Verification items for this drawing (mm, ordinates from the low corner). A direction names the side the tool comes from. Give positions to 0.01 mm unless a question says otherwise; leave off trailing zeros. Order: outer loops, then holes, each group sorted by start corner. A loop starts at its lowest first (then second) coordinate and runs counter-clockwise, first axis right, second up. Notation, with made-up numbers: M 78,49.5 L 83,49.5 A26 cw 83,64.5 Z; hole C -14,84 d9. An arc over 180 degrees is marked long. Answer as a JSON object with one key per item and string values.
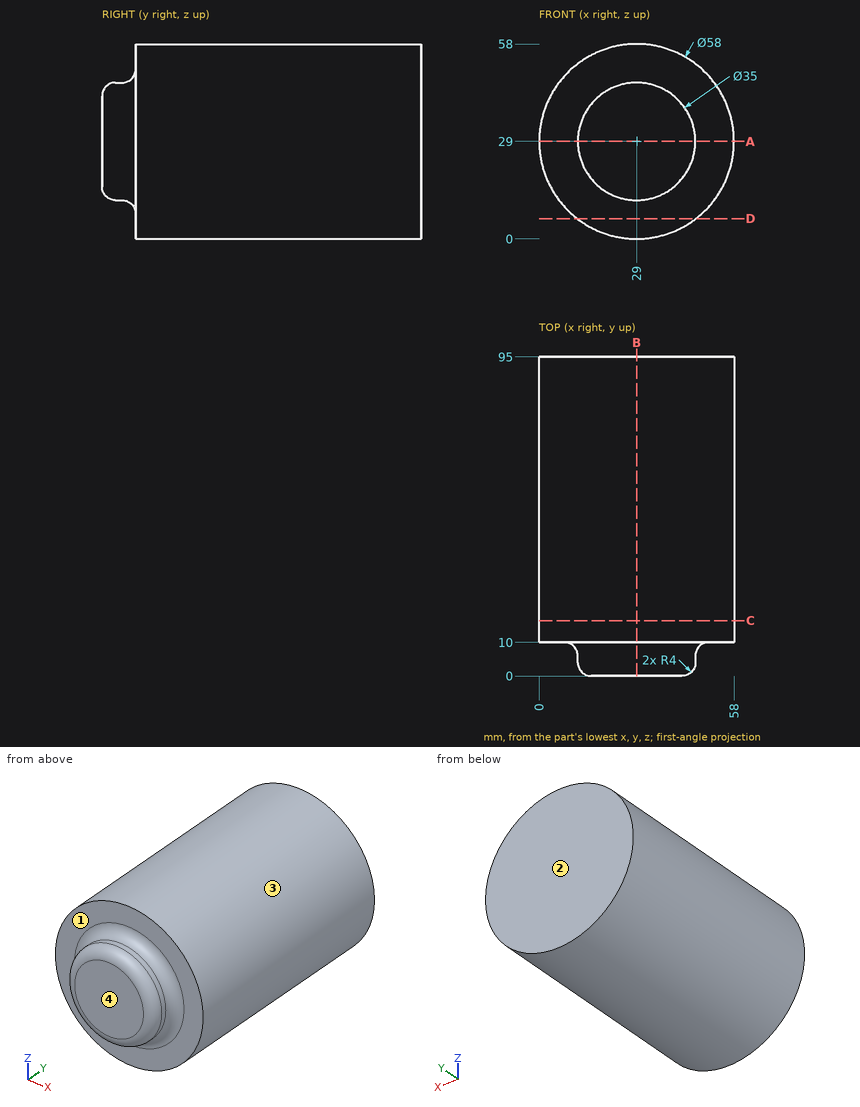
Q1. Gauge pin test, flat ends, axial feed: pin 1 Ø2 at (y, z) = (84, 40.5) entering from -X; pin 2 Ø5 at (x, y) = (15, 51) entering from +Z; pin 3 Ø3 at (x, y) = (34, 37.5) entering from -Z. Record the tip position at first contact, or that the pin passes through.
Resolved:
{"pin 1": "stops at x = 1.97", "pin 2": "stops at z = 55.62", "pin 3": "stops at z = 0.21"}
Q2. Section check B-B on x = 29. Record the cut outline in (y, z).
Resolved:
{"outline": "M 0,15.5 A4 ccw 4,11.5 L 6,11.5 A4 cw 10,7.5 L 10,0 L 95,0 L 95,58 L 10,58 L 10,50.5 A4 cw 6,46.5 L 4,46.5 A4 ccw 0,42.5 Z"}
Q3. Tool access check on the marked faces 1 and 2. Record the directions out of +Z, -Z, +X, -X, +Y, -Y that give a thin tool (end or side, any length) a straight path to the whole face; none if there is none.
Resolved:
{"face 1": "-Y", "face 2": "+Z, -Z, +X, -X, +Y"}
Q4. Section check D-D on z = 6. Record the cut outline in (x, y), then the cut area to 3 significant figures.
Resolved:
{"outline": "M 11.34,10 L 46.66,10 L 46.66,95 L 11.34,95 Z", "area": "3,000 mm²"}
Q5. Release check for a two-part mould opening along Z. For the marked faces 3 and 4 record: +Z half, -Z half, draft (parallel to the pull), parting line (faces both ways), or undercut.
Resolved:
{"face 3": "parting line", "face 4": "draft"}
Q6. Section check A-A on z = 29. Record the cut outline in (x, y).
Resolved:
{"outline": "M 0,10 L 7.5,10 A4 cw 11.5,6 L 11.5,4 A4 ccw 15.5,0 L 42.5,0 A4 ccw 46.5,4 L 46.5,6 A4 cw 50.5,10 L 58,10 L 58,95 L 0,95 Z"}
Q7. Section check C-C on y = 16.5. Record the cut outline in (x, z), then the cut area to 3 significant figures.
Resolved:
{"outline": "C 29,29 d58", "area": "2,640 mm²"}
Q8. Material ranges on L1, parallel to Y at x = 3, z = 24.5; L2, parallel to Z at x = 29.5, y = 28; L3, parallel to Y at x = 27.5, z = 42.5, recorded low to high.
Resolved:
{"L1": "y = 10 to 95", "L2": "z = 0 to 58", "L3": "y = 0 to 95"}
